Read the model definition and answer for the solid it produces. Units are mm, in the model's axes. Face numbers are marked on the shaded views. A direction names the side the tool comes from. Coordinates: 2 decimals unless noted, no trailing zeros. Write each loop counter-clockwise with the first axis right and the second up, starting at its lowest first coordinate (ties: lowest second). Pieces come first, ordered by that corner, then holes. Notation, with made-up numbers: (20, -40) -> (47, -40) arc R20 cw to (47, -19) -> close; hole circle Ø6 at (36, -38). An arc over 180 degrees is marked (long way). Return JSON: item names as keys, results as strings.
from build123d import *

# Parameters (mm, degrees)
SKETCH1_R           = 28.5
SKETCH1_R_2         = 15
BOSS_EXTRUDE1_DEPTH = 38
SKETCH2_W           = 57
SKETCH2_H           = 84
BOSS_EXTRUDE2_DEPTH = 16
SKETCH6_W           = 57
SKETCH6_H           = 38
BOSS_EXTRUDE4_DEPTH = 14
SKETCH7_W           = 57
SKETCH7_H           = 38
BOSS_EXTRUDE5_DEPTH = 14
SKETCH8_R           = 8
CUT_EXTRUDE3_DEPTH  = 104.847243584
CUT_EXTRUDE4_DEPTH  = 104.847243584
CUT_EXTRUDE5_START  = -38
CUT_EXTRUDE5_DEPTH  = 38
ESCALA1_SCALE       = 0.5


with BuildPart() as part:
    # Sketch1 → Boss-Extrude1 (new body)
    with BuildSketch(Plane(origin=(0, 0, 0), x_dir=(1, 0, 0), z_dir=(0, 1, 0))):
        with Locations(Location((0, 0, 0), (0, 0, 270))):
            Circle(SKETCH1_R)
        with Locations(Location((0, 0, 0), (0, 0, 270))):
            Circle(SKETCH1_R_2, mode=Mode.SUBTRACT)
    extrude(amount=BOSS_EXTRUDE1_DEPTH)

    # Sketch2 → Boss-Extrude2 (add)
    with BuildSketch(Plane.XZ):
        Rectangle(SKETCH2_W, SKETCH2_H)
    extrude(amount=BOSS_EXTRUDE2_DEPTH)

    # Sketch6 → Boss-Extrude4 (add)
    with BuildSketch(Plane.XY.offset(42)):
        with Locations((0, -35)):
            Rectangle(SKETCH6_W, SKETCH6_H)
    extrude(amount=-BOSS_EXTRUDE4_DEPTH)

    # Sketch7 → Boss-Extrude5 (add)
    with BuildSketch(Plane(origin=(0, 0, -42), x_dir=(-1, 0, 0), z_dir=(0, 0, -1))):
        with Locations((0, -35)):
            Rectangle(SKETCH7_W, SKETCH7_H)
    extrude(amount=-BOSS_EXTRUDE5_DEPTH)

    # Sketch8 → Cut-Extrude3 (cut, through all)
    with BuildSketch(Plane(origin=(0, 0, -42), x_dir=(-1, 0, 0), z_dir=(0, 0, -1))):
        with Locations((0, -34)):
            Circle(SKETCH8_R)
    extrude(amount=-CUT_EXTRUDE3_DEPTH, mode=Mode.SUBTRACT)

    # Sketch9 → Cut-Extrude4 (cut, through all)
    with BuildSketch(Plane.XY.offset(42)):
        with BuildLine():
            Line((-19.473528625, -38.558693112), (-28.5, 0))
            Line((-28.5, 0), (-28.5, -54))
            Line((-28.5, -54), (0, -54))
            ThreePointArc((0, -54), (-12.42630552, -49.671213454), (-19.473528625, -38.558693112))
        make_face()
        with BuildLine():
            ThreePointArc((19.473522225, -38.558720453), (12.426294519, -49.671222177), (0, -54))
            Line((0, -54), (28.5, -54))
            Line((28.5, -54), (28.5, 0))
            Line((28.5, 0), (19.473522225, -38.558720453))
        make_face()
    extrude(amount=-CUT_EXTRUDE4_DEPTH, mode=Mode.SUBTRACT)

    # Sketch11 → Cut-Extrude5 (cut)
    with BuildSketch(Plane(origin=(0, 38, 0), x_dir=(1, 0, 0), z_dir=(0, 1, 0)).offset(CUT_EXTRUDE5_START)):
        with BuildLine():
            Line((-4, 17.956832295), (4, 17.956832295))
            Line((4, 17.956832295), (4, 14.456832295))
            ThreePointArc((4, 14.456832295), (0, 15), (-4, 14.456832295))
            Line((-4, 14.456832295), (-4, 17.956832295))
        make_face()
    extrude(amount=CUT_EXTRUDE5_DEPTH, mode=Mode.SUBTRACT)


with BuildPart() as part_1:
    # Escala1: scaled about (0, -2.092250253, 0.088985483)
    add(part.part.scale(ESCALA1_SCALE).moved(Location((0, -1.046125127, 0.044492742))))


solid = part_1.part
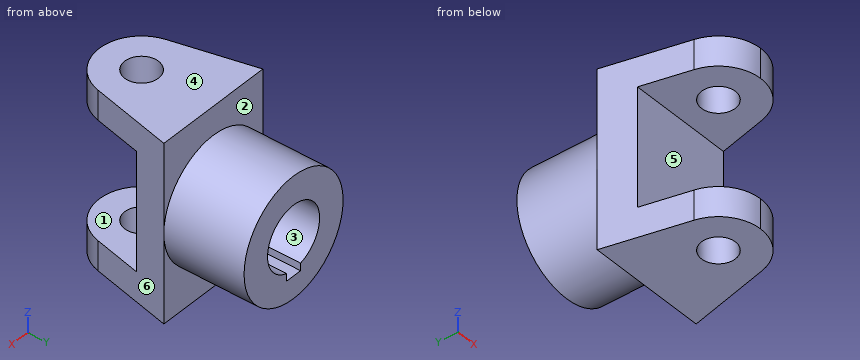
1. The part is cut by section B-B (y = 2.5). Determine the outline of the cut face in (x, z), then the cut area to 3 significant figures.
Taken from the geometry:
{"outline": "circle Ø28.5 at (0, 0.04); hole (-2, -8.93) -> (2, -8.93) -> (2, -7.18) arc R7.5 ccw (long way) to (-2, -7.18) -> close", "area": "455 mm2"}
2. A tool of negligible diameter and unlimited length cuts with its end or side. For the marked faces 1, 2 and 3, from which of +Z, -Z, +X, -X, +Y, -Y can it reach the whole face along a straight path? Write none if from no direction.
Taken from the geometry:
{"face 1": "+X, -X, -Y", "face 2": "+Z, +Y", "face 3": "+Y"}
3. Flat-ended cylindrical pins translate along their axes: pin 1 Ø1.4 at (y, z) = (10, -8) entering from +X; pin 2 Ø1.4 at (y, z) = (6, -8) entering from -X; pin 3 Ø1.2 at (x, y) = (-0.5, 8) entering from +Z; pin 4 Ø5 at (y, z) = (-14.5, 9.5) entering from -X. Find the tip coordinate at first contact, or state that the pin passes through.
Taken from the geometry:
{"pin 1": "stops at x = 12.21", "pin 2": "stops at x = -12.21", "pin 3": "stops at z = 14.29", "pin 4": "passes through"}
4. The part is cut by section C-C (x = -1). Determine the outline of the cut face in (y, z).
Taken from the geometry:
{"outline": "(-28, -20.96) -> (-21.92, -20.96) -> (-21.92, -13.96) -> (-28, -13.96) -> close; (-28, 14.04) -> (-21.92, 14.04) -> (-21.92, 21.04) -> (-28, 21.04) -> close; (-14.17, -20.96) -> (-1.05, -20.96) -> (-1.05, -14.17) -> (17.95, -14.17) -> (17.95, -8.93) -> (-1.05, -8.93) -> (-1.05, 7.48) -> (17.95, 7.48) -> (17.95, 14.26) -> (-1.05, 14.26) -> (-1.05, 21.04) -> (-14.17, 21.04) -> (-14.17, 14.04) -> (-9.05, 14.04) -> (-9.05, -13.96) -> (-14.17, -13.96) -> close"}
5. Consider L1, parallel to Y at x = 0, z = -17; L2, parallel to Z at x = -4.75, y = -14.5; L3, parallel to Y at x = 9.25, z = -11. Determine where each line is inside the solid, lowest interval first.
Taken from the geometry:
{"L1": "y = -28.05 to -22.05, -14.05 to -1.05", "L2": "z = -20.96 to -13.96, 14.04 to 21.04", "L3": "y = -9.05 to -1.05"}
6. For a pull along Z with two mould halves and no side action, classify the marked faces 4, 5 and 6 as +Z half, -Z half, draft (parallel to the pull), parting line (faces both ways), or undercut.
Taken from the geometry:
{"face 4": "+Z half", "face 5": "undercut", "face 6": "draft"}
7. The part is cut by section A-A (y = -19.5). Determine the outline of the cut face in (x, z).
Taken from the geometry:
{"outline": "(-9.93, -20.96) -> (-3.73, -20.96) -> (-3.73, -13.96) -> (-9.93, -13.96) -> close; (-9.93, 14.04) -> (-3.73, 14.04) -> (-3.73, 21.04) -> (-9.93, 21.04) -> close; (3.73, -20.96) -> (9.93, -20.96) -> (9.93, -13.96) -> (3.73, -13.96) -> close; (3.73, 14.04) -> (9.93, 14.04) -> (9.93, 21.04) -> (3.73, 21.04) -> close"}
8. The part is cut by section D-D (z = -6.5). Determine the outline of the cut face in (x, y), then the cut area to 3 significant figures.
Taken from the geometry:
{"outline": "(-14.25, -1.05) -> (-12.38, -9.05) -> (12.38, -9.05) -> (14.25, -1.05) -> (12.66, -1.05) -> (12.66, 17.95) -> (3.66, 17.95) -> (3.66, -1.05) -> (-3.66, -1.05) -> (-3.66, 17.95) -> (-12.66, 17.95) -> (-12.66, -1.05) -> close", "area": "555 mm2"}
